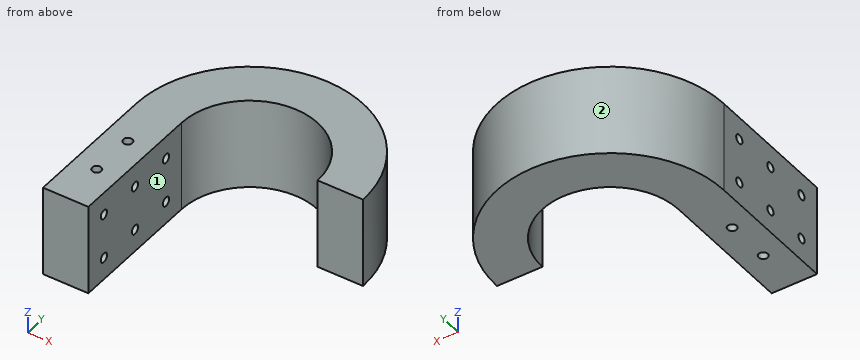
from build123d import *

# Parameters (mm, degrees)
BOSS_EXTRUDE1_DEPTH    = 50.8
F_10_CLEARANCE_HOLE1_D = 5.1054
F_10_CLEARANCE_HOLE2_D = 5.1054


with BuildPart() as part:
    # Sketch1 → Boss-Extrude1 (new body)
    with BuildSketch(Plane.XY):
        with BuildLine():
            Line((101.6, 76.2), (127, 76.2))
            ThreePointArc((127, 76.2), (63.5, 139.7), (0, 76.2))
            Line((0, 76.2), (0, 0))
            Line((0, 0), (25.4, 0))
            Line((25.4, 0), (25.4, 76.2))
            ThreePointArc((25.4, 76.2), (63.5, 114.3), (101.6, 76.2))
        make_face()
    extrude(amount=BOSS_EXTRUDE1_DEPTH)

    # #10 Clearance Hole1 (through all)
    with Locations(Plane.XY.offset(50.8)):
        with Locations((12.7, 50.8), (12.7, 25.4)):
            Hole(F_10_CLEARANCE_HOLE1_D / 2)

    # #10 Clearance Hole2 (through all)
    with Locations(Plane.ZY):
        with Locations((12.7, 38.1), (12.7, 12.7), (12.7, 63.5), (38.1, 63.5), (38.1, 12.7), (38.1, 38.1)):
            Hole(F_10_CLEARANCE_HOLE2_D / 2)


solid = part.part
Input: part model. Units: mm. Frame: model coordinates. Face numbers are marked on the shaded views. A direction names the side the tool comes from. Give positions to 0.01 mm unless a question says otherwise; leave off trailing zeros. Write each loop counter-clockwise with the first axis right and the second up, starting at its lowest first coordinate (ties: lowest second). Pieces come first, ordered by that corner, then holes. Notation, with made-up numbers: M 88.25,48.25 L 124.25,48.25 A23 cw 124.25,82.25 Z; hole C 57.5,-6.5 d8. An arc over 180 degrees is marked long. Write item = value, one per line. Start each with the question number.
1) First-contact query: pin 1 Ø1.5 at (x, z) = (93, 19) entering from -Y; pin 2 Ø8 at (y, z) = (91.5, 13) entering from +X; pin 3 Ø8 at (y, z) = (63.5, 12.7) entering from +X. Flat tips, straight axial feed; report the tip coordinate or a pass-through.
2) Cut plane D-D on y = 94.5. Return the cut outline in (x, z), then the cut area to 3 significant figures.
3) Cut plane C-C on y = 38.1. Return the cut outline in (x, z).
4) Cut plane A-A on x = 12.7. Count the separate pieces of the cut face and the enclosed holes in it, then the cut area to 3 significant figures.
5) Reachability of the marked faces 1 and 2 from +Z, -Z, +X, -X, +Y, -Y: full face, straight path, thin tool, end or side. Return the list, or none.
6) Material intervals for line 1 along Y through (x, z) = (12.7, 32.5); line 2 along Y through (x, z) = (11, 38.1); line 3 along Y through (x, z) = (19, 12.7), sorted ascending. Write a range as [from, to].
7) Cut plane B-B on z = 38.1. Return the cut outline in (x, y), then the cut area to 3 significant figures.
Solved:
q1.pin_1 = 99.36
q1.pin_2 = 125.99
q1.pin_3 = 25.4
q2.outline = M 2.69,0 L 30.08,0 L 30.08,50.8 L 2.69,50.8 Z; M 96.92,0 L 124.31,0 L 124.31,50.8 L 96.92,50.8 Z
q2.area = 2,780 mm2
q3.outline = M 0,0 L 25.4,0 L 25.4,10.15 L 0,10.15 Z; M 0,15.25 L 25.4,15.25 L 25.4,35.55 L 0,35.55 Z; M 0,40.65 L 25.4,40.65 L 25.4,50.8 L 0,50.8 Z
q4.separate_pieces = 3
q4.enclosed_holes = 6
q4.area = 5,160 mm2
q5.face_1 = +Z, -Z, +X, -Y
q5.face_2 = +Z, -Z, +Y
q6.line_1 = [0, 22.85], [27.95, 48.25], [53.35, 114.3]
q6.line_2 = [0, 10.15], [15.25, 23.5], [27.3, 35.55], [40.65, 48.9], [52.7, 60.95], [66.05, 111.92]
q6.line_3 = [0, 10.15], [15.25, 35.55], [40.65, 60.95], [66.05, 121.5]
q7.outline = M 0,0 L 25.4,0 L 25.4,10.15 L 0,10.15 Z; M 0,15.25 L 25.4,15.25 L 25.4,35.55 L 0,35.55 Z; M 0,40.65 L 25.4,40.65 L 25.4,60.95 L 0,60.95 Z; M 0,66.05 L 25.4,66.05 L 25.4,76.2 A38.1 cw 101.6,76.2 L 127,76.2 A63.5 ccw 0,76.2 Z; hole C 12.7,25.4 d5.11; hole C 12.7,50.8 d5.11
q7.area = 5,560 mm2
